Geometry check sheet. Reference: the model listing, model coordinates, mm. Face numbers are marked on the shaded views. A direction names the side the tool comes from. Coordinates: 2 decimals unless noted, no trailing zeros. Write each loop counter-clockwise with the first axis right and the second up, starting at its lowest first coordinate (ties: lowest second). Pieces come first, ordered by that corner, then holes. Notation, with made-up numbers: (-36, -27) -> (22, -27) arc R21 cw to (22, 11) -> close; hole circle Ø6 at (14.5, -30.75). An arc over 180 degrees is marked (long way). One line per question, with ' | ' between items.
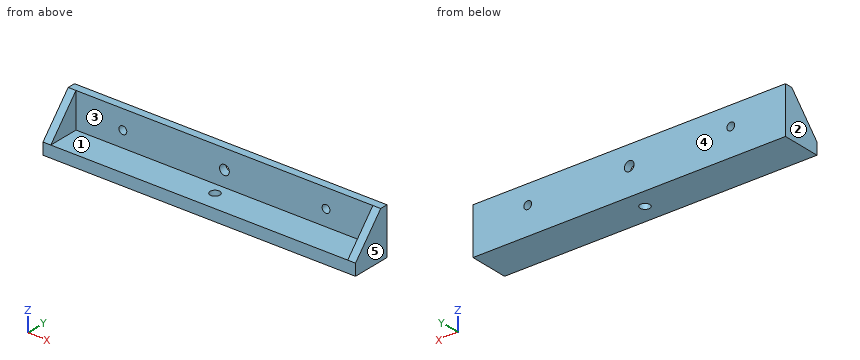
from build123d import *

# Parameters (mm, degrees)
F0_W      = 80
F0_H      = 10
F1_DEPTH  = 3
F2_W      = 80
F2_H      = 2
F3_DEPTH  = 9
F4_R      = 1.25
F5_DEPTH  = 3.001
F6_R      = 1.25
F7_DEPTH  = 2.001
F9_DEPTH  = 2
F10_R     = 1
F11_DEPTH = 2.001


# Not quite as in the source:
# - a pattern or mirror of a feature is missing from the dataset's text; its kind, count and spacing are read off the source's solid


with BuildPart() as f1:
    # F0 (on Top) → F1 (new body)
    with BuildSketch(Plane.XY):
        Rectangle(F0_W, F0_H)
    extrude(amount=F1_DEPTH)

    # F2 (on face) → F3 (join)
    with BuildSketch(Plane.XY.offset(3)):
        with Locations((0, 4)):
            Rectangle(F2_W, F2_H)
    extrude(amount=F3_DEPTH)

    # F4 (on face) → F5 (cut, through all)
    with BuildSketch(Plane.XY.offset(3)):
        Circle(F4_R)
    extrude(amount=-F5_DEPTH, mode=Mode.SUBTRACT)

    # F6 (on face) → F7 (cut, through all)
    with BuildSketch(Plane.XZ.offset(-3)):
        with Locations((0, 7)):
            Circle(F6_R)
    extrude(amount=-F7_DEPTH, mode=Mode.SUBTRACT)

    # F8 (on face) → F9 (join)
    with BuildSketch(Plane(origin=(-40, 0, 0), x_dir=(0, -1, 0), z_dir=(-1, 0, 0))):
        Polygon((5, 3), (-3, 12), (-3, 3), align=None)
    f9 = extrude(amount=-F9_DEPTH)

    # F9_copies: F9 across plane
    add(f9.mirror(Plane(origin=(0, 0, 0), x_dir=(0, 0, 1), z_dir=(1, 0, 0))))

    # F10 (on face) → F11 (cut, through all)
    with BuildSketch(Plane.XZ.offset(-3)):
        with Locations((-26, 7.0934407413)):
            Circle(F10_R)
        with Locations((26, 7.0934407413)):
            Circle(F10_R)
    extrude(amount=-F11_DEPTH, mode=Mode.SUBTRACT)


solid = f1.part
1. Cross-section at A-A on x = 0. Record the boundary of the cut face in (y, z).
Worked answers:
outline: (-5, 0) -> (-1.25, 0) -> (-1.25, 3) -> (-5, 3) -> close; (1.25, 0) -> (5, 0) -> (5, 5.75) -> (3, 5.75) -> (3, 3) -> (1.25, 3) -> close; (3, 8.25) -> (5, 8.25) -> (5, 12) -> (3, 12) -> close
2. Cross-section at B-B on x = -26. Record the boundary of the cut face in (y, z).
Worked answers:
outline: (-5, 0) -> (5, 0) -> (5, 6.09) -> (3, 6.09) -> (3, 3) -> (-5, 3) -> close; (3, 8.09) -> (5, 8.09) -> (5, 12) -> (3, 12) -> close
3. Cross-section at D-D on z = 9.25. Record the boundary of the cut face in (x, y).
Worked answers:
outline: (-40, 0.56) -> (-38, 0.56) -> (-38, 3) -> (38, 3) -> (38, 0.56) -> (40, 0.56) -> (40, 5) -> (-40, 5) -> close
4. Mould release check, pull along X, two halves, no side actions. Record for the marked faces 3, 4 and 5: released by +X, released by -X, zero draft, split by the parting line, or undercut.
Worked answers:
face 3: undercut | face 4: zero draft | face 5: released by +X
5. Cross-section at C-C on y = -3.25. Record the boundary of the cut face in (x, z), and give its area (3 significant figures).
Worked answers:
outline: (-40, 0) -> (40, 0) -> (40, 4.97) -> (38, 4.97) -> (38, 3) -> (-38, 3) -> (-38, 4.97) -> (-40, 4.97) -> close | area: 248 mm²
6. Go/stop test with flat-tipped pins: P1, Ø1.5, axis at x = 0, y = 0, coming from the +Z side; P2, Ø5, axis at x = 9.5, z = 8, coming from the -Y side; P3, Ø6, axis at x = -28, y = -1, coming from the +Z side. Record where each tip stops, or that it passes through.
Worked answers:
P1: through | P2: y = 3 | P3: z = 3
7. Tool access check on the marked faces 1 and 2. Record the directions out of +Z, -Z, +X, -X, +Y, -Y that give a thin tool (end or side, any length) a straight path to the whole face; none if there is none.
Worked answers:
face 1: +Z, -Y | face 2: +Z, -Z, -X, +Y, -Y
8. Material ranges on line 1 (X direction, y = 2, z = 7); line 2 (Z direction, x = 0, y = 4.2); line 3 (X direction, y = 4.25, z = 7.5), recorded low to high. Write a range as from..to.
Worked answers:
line 1: -40..-38, 38..40 | line 2: 0..5.75, 8.25..12 | line 3: -40..-26.91, -25.09..-1.15, 1.15..25.09, 26.91..40
